from build123d import *

# Parameters (mm, degrees)
F1_DEPTH = 10.922
F2_W     = 52.578
F2_H     = 10.922
F3_DEPTH = 33.528
F5_DEPTH = 10.923
F7_DEPTH = 115.7693519126
F8_R     = 7.874
F9_DEPTH = 10.923


# Not quite as in the source:
# - a feature names something its author has since deleted; it is built from what else it names


with BuildPart() as f1:
    # F0 (on Front) → F1 (new body)
    with BuildSketch(Plane.XZ):
        Polygon((-14.4320207924, 31.8836830556), (-46.1820207924, 31.8836830556), (-46.1820207924, -27.459501562), (-34.950372705, -27.459501562), (69.5863311203, -27.459501562), (69.5863311203, 9.3710335113), align=None)
    extrude(amount=-F1_DEPTH)

    # F2 (on face) → F3 (join)
    with BuildSketch(Plane.XZ):
        with Locations((-8.9710207924, -21.998501562)):
            Rectangle(F2_W, F2_H)
        Polygon((-35.2600207924, 23.340498438), (-46.1820207924, 23.340498438), (-46.1820207924, -27.459501562), (-35.2600207924, -27.459501562), (-35.2600207924, -16.537501562), align=None)
    extrude(amount=F3_DEPTH)

    # F4 (on face) → F5 (cut, through all)
    with BuildSketch(Plane.XY.offset(-16.537501562)):
        Polygon((17.3179792076, -33.528), (17.3179792076, 0), (-35.2600207924, -33.528), align=None)
    extrude(amount=-F5_DEPTH, mode=Mode.SUBTRACT)

    # F6 (on face) → F7 (cut, through all)
    with BuildSketch(Plane(origin=(-46.1820207924, 0, 0), x_dir=(0, -1, 0), z_dir=(-1, 0, 0))):
        Polygon((16.9568925737, 23.340498438), (33.528, -5.361501562), (33.528, 23.340498438), align=None)
    extrude(amount=-F7_DEPTH, mode=Mode.SUBTRACT)

    # F8 (on face) → F9 (cut, through all)
    with BuildSketch(Plane.XZ):
        with Locations((50.5363311203, -8.409501562)):
            Circle(F8_R)
    extrude(amount=-F9_DEPTH, mode=Mode.SUBTRACT)


solid = f1.part
Check sheet for the modelled part. Datum: model origin and axes. Units: mm. A direction names the side the tool comes from. Give positions to 0.01 mm unless a question says otherwise; leave off trailing zeros. Loops run counter-clockwise (first coordinate to the right, second up) from the corner with the lowest first, then second, coordinate; pieces in that order, holes last. Notation, with made-up numbers: M -0.75,16.25 L 39.25,16.25 A17 cw 39.25,47.25 Z; hole C -16.75,44 d9. An arc over 180 degrees is marked long. Answer as a JSON object with one key per item and string values. Group by question number.
Q1. Material ranges on line 1 along Z through (x, y) = (-11, -2); line 2 along Y through (x, z) = (25, 1); line 3 along X through (y, z) = (-20.5, 1.5), recorded low to high. Write a range as [from, to].
Q2. Cross-section at A-A on x = 50. Record the cut outline in (y, z), then the cut area to 3 significant figures.
Q3. Release check for a two-part mould opening along X. For faces 4 (the flat face through (-35.26, -13, 3)), 5 (the cylindrical face through (44.73, 5.38, -3.09)), 6 (the flat face through (-41, -33.528, -16)) record: released by +X, released by -X, zero draft, split by the parting line, or undercut.
Q4. Cross-section at D-D on z = -7. Record the cut outline in (x, y).
Q5. Go/stop test with flat-tipped pins: P1, Ø17, axis at y = -24, z = 9.5, coming from the +X side; P2, Ø25, axis at x = 50.54, z = -8.41, coming from the -Y side; P3, Ø2, axis at x = -3.5, y = -15.5, coming from the -Z side; P4, Ø10, axis at x = -32, z = 22, coming from the -Y side. Record where each tip stops, or that it passes through.
Q6. Access from +Z, -Z, +X, -X, +Y, -Y to the whole of each face (thin tool, end or side, straight path). Record for faces 1 (the flat face through (-15, -13, -16.538)), 2 (the flat face through (-41, -8, 23.34)), 3 (the flat face through (-8.603, -16.529, -21.922)).
Q7. Cross-section at C-C on y = 8.5. Record the cut outline in (x, z), then the cut area to 3 significant figures.
Q8. Cross-section at B-B on z = -24. Record the cut outline in (x, y), then the cut area to 3 significant figures.
Evaluation:
{
 "1": {"line 1": "z = [-27.46, -16.54]", "line 2": "y = [0, 10.92]", "line 3": "x = [-46.18, -35.26]"},
 "2": {"outline": "M 0,-27.46 L 10.92,-27.46 L 10.92,-16.27 L 0,-16.27 Z; M 0,-0.55 L 10.92,-0.55 L 10.92,14.62 L 0,14.62 Z", "area": "288 mm2"},
 "3": {"face 4": "released by +X", "face 5": "undercut", "face 6": "zero draft"},
 "4": {"outline": "M -46.18,-33.53 L -35.26,-33.53 L -35.26,0 L 42.79,0 L 42.79,10.92 L -46.18,10.92 Z; M 58.28,0 L 69.59,0 L 69.59,10.92 L 58.28,10.92 Z"},
 "5": {"P1": "stops at x = -35.26", "P2": "stops at y = 0", "P3": "passes through", "P4": "stops at y = -19.92"},
 "6": {"face 1": "+Z, +X, -Y", "face 2": "+Z, +X, -X, -Y", "face 3": "+Z, -Z, +X, -Y"},
 "7": {"outline": "M -46.18,-27.46 L 69.59,-27.46 L 69.59,9.37 L -14.43,31.88 L -46.18,31.88 Z; hole C 50.54,-8.41 d15.75", "area": "5,730 mm2"},
 "8": {"outline": "M -46.18,-33.53 L -35.26,-33.53 L 17.32,0 L 69.59,0 L 69.59,10.92 L -46.18,10.92 Z", "area": "2,510 mm2"}
}
